The listing builds one solid part. Answer for the finished solid, in the listing's coordinates (mm). Face numbers are marked on the shaded views. A direction names the side the tool comes from. Give positions to 0.01 mm unless a question says otherwise; leave off trailing zeros. Order: outer loops, then holes, each group sorted by start corner. A loop starts at its lowest first (then second) coordinate and runs counter-clockwise, first axis right, second up. Notation, with made-up numbers: (-40, 39.25) - (10, 39.25) arc R30 cw to (10, 65.25) - close; hole circle Ø1 at (-3, 26). An arc over 180 degrees is marked (long way). Answer in a Markdown table with one row per item. Add a question column.
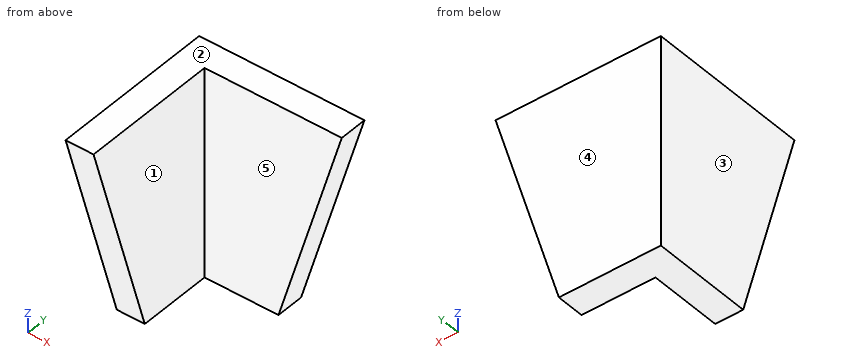
```python
from build123d import *

# Parameters (mm, degrees)
BOSS_EXTRUDE1_DEPTH = 30
CUT_EXTRUDE1_DEPTH  = 10
CUT_EXTRUDE2_DEPTH  = 83.096264686


with BuildPart() as part:
    # Sketch1 → Boss-Extrude1 (new, symmetric)
    with BuildSketch(Plane.XY):
        Polygon((40, 0), (0, 0), (0, -40), (-8, -40), (-8, 8), (40, 8), align=None)
    extrude(amount=BOSS_EXTRUDE1_DEPTH, both=True)

    # Sketch2 → Cut-Extrude1 (cut)
    with BuildSketch(Plane.XZ):
        Polygon((39.240243059, 30), (21.129361647, -30), (40, -30), (40, 30), align=None)
    extrude(amount=-CUT_EXTRUDE1_DEPTH, mode=Mode.SUBTRACT)

    # Sketch4 → Cut-Extrude2 (cut, through all)
    with BuildSketch(Plane(origin=(0, 0, -30), x_dir=(-1, 0, 0), z_dir=(0, 0, -1))):
        Polygon((0, 0), (8, 8), (8, -40), (0, -40), align=None)
    extrude(amount=-CUT_EXTRUDE2_DEPTH, mode=Mode.SUBTRACT)

    # Mirror1: part across plane


with BuildPart() as part_1:
    add(part.part)
    add(part.part.mirror(Plane(origin=(0, 0, 30), x_dir=(0, 0, 1), z_dir=(0.7071067811865476, 0.7071067811865476, 0))))


solid = part_1.part
```
(1) Straight lines are drawn through the part: line 1 (X direction, y = -15, z = 18.5); line 2 (Y direction, x = 9.5, z = 26.5); line 3 (X direction, y = 4, z = -20.5). For each, find the intervals that lie inside material, in ascending order.
(2) Find section B-B, the plane y = -2. Write down the section's boundary in (x, z), plus the area to 3 significant figures.
(3) For the marked faces 4 and 5, determine the directions among +Z, -Z, +X, -X, +Y, -Y from which every point of the face is accessible in a straight line to the end or side of a thin tool.
(4) Find section A-A, the plane x = -5. Write down the section's boundary in (y, z), plus the area to 3 significant figures.
(5) Find section D-D, the plane z = -23.5. Write down the section's boundary in (x, y).
(6) Each of these flat-tipped pins is pushed along its axis until it touches: P1, Ø1.5, axis at x = 10, z = 3.5, coming from the -Y side; P2, Ø12, axis at x = 4, y = -18.5, coming from the +Z side; P3, Ø5, axis at y = -29, z = 7.5, coming from the +X side. Where does it stop, or does it pass through?
(7) The mould has two halves that part along X. Classify the marked faces 1, 2 and 3: +X half, -X half, draft (parallel to the pull), parting line (faces both ways), or undercut.
(8) Find section C-C, the plane z = -17. Write down the section's boundary in (x, y), plus the area to 3 significant figures.
Answer key:
| question | item | result |
|---|---|---|
| 1 | line 1 | -8 to 0 |
| 1 | line 2 | 0 to 8 |
| 1 | line 3 | -8 to 24 |
| 2 | outline | (-8, -30) - (0, -30) - (0, 30) - (-8, 30) - close |
| 2 | area | 480 mm² |
| 3 | face 4 | +Z, -Z, +X, -X, +Y |
| 3 | face 5 | +Z, -Z, +X, -Y |
| 4 | outline | (-39.24, 30) - (-21.13, -30) - (8, -30) - (8, 30) - close |
| 4 | area | 2,290 mm² |
| 5 | outline | (-8, -23.09) - (0, -23.09) - (0, 0) - (23.09, 0) - (23.09, 8) - (-8, 8) - close |
| 6 | P1 | y = 0 |
| 6 | P2 | z = 30 |
| 6 | P3 | x = 0 |
| 7 | face 1 | +X half |
| 7 | face 2 | draft |
| 7 | face 3 | -X half |
| 8 | outline | (-8, -25.05) - (0, -25.05) - (0, 0) - (25.05, 0) - (25.05, 8) - (-8, 8) - close |
| 8 | area | 465 mm² |
